The model under review builds one solid part; all positions refer to its coordinate system, in mm. Round coordinates to 2 decimals unless told otherwise and drop trailing zeros. Loops run counter-clockwise (first coordinate to the right, second up) from the corner with the lowest first, then second, coordinate; pieces in that order, holes last. Notation, with made-up numbers: M -13.5,-28.5 L 7.5,-28.5 A22 ccw 7.5,-14.5 Z; hole C -33,37.25 d5. An arc over 180 degrees is marked long. Return JSON: item names as keys, results as strings. Group by question number.
Q1. Consider section A-A (x = 0). State the section outline as (y, z) points (3 decimals).
Q2. Consider section B-B (z = 44.45). State the section outline as (x, y) points, and give its area (3 significant figures).
Q3. To check wall thickness, follow line 1 along Z through (x, y) = (0, 8); line 2 along X through (y, z) = (21.5, 44.45); line 3 along X through (y, z) = (16, 44). State the ranges of each line that lie inside material, in increasing order.
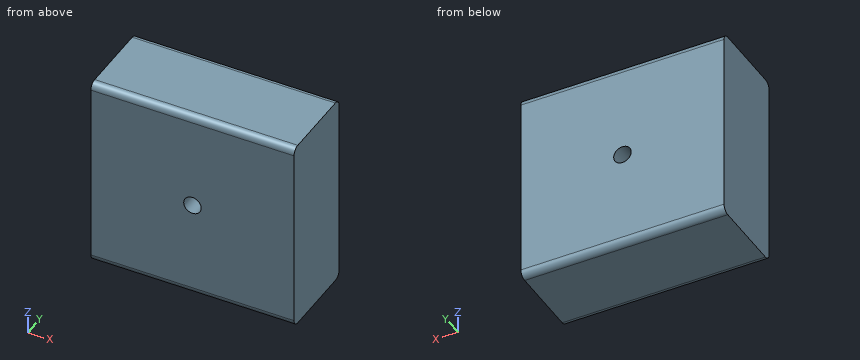
from build123d import *

# Parameters (mm, degrees)
SKETCH1_W                      = 92.075
SKETCH1_H                      = 38.1
BOSS_EXTRUDE1_DEPTH            = 88.9
FILLET1_R                      = 3.175
F_5_16_0_3125_DIAMETER_HOLE1_D = 7.9375


with BuildPart() as part:
    # Sketch1 → Boss-Extrude1 (new body)
    with BuildSketch(Plane.XY):
        with Locations((0, 19.05)):
            Rectangle(SKETCH1_W, SKETCH1_H)
    extrude(amount=BOSS_EXTRUDE1_DEPTH)

    # Fillet1
    fillet1_edges = [part.edges().sort_by_distance(p)[0] for p in [
        (0, 38.1, 88.9),
        (0, 38.1, 0),
        (0, 0, 0),
        (0, 0, 88.9),
    ]]
    fillet(fillet1_edges, radius=FILLET1_R)

    # 5/16 (0.3125) Diameter Hole1 (through all)
    with Locations(Plane(origin=(0, 38.1, 0), x_dir=(1, 0, 0), z_dir=(0, 1, 0))):
        with Locations((0, -44.45)):
            Hole(F_5_16_0_3125_DIAMETER_HOLE1_D / 2)


solid = part.part
Values:
{
 "1": {"outline": "M 0,3.175 A3.175 ccw 3.175,0 L 34.925,0 A3.175 ccw 38.1,3.175 L 38.1,40.481 L 0,40.481 Z; M 0,48.419 L 38.1,48.419 L 38.1,85.725 A3.175 ccw 34.925,88.9 L 3.175,88.9 A3.175 ccw 0,85.725 Z"},
 "2": {"outline": "M -46.04,0 L -3.97,0 L -3.97,38.1 L -46.04,38.1 Z; M 3.97,0 L 46.04,0 L 46.04,38.1 L 3.97,38.1 Z", "area": "3,210 mm2"},
 "3": {"line 1": "z = 0 to 40.48, 48.42 to 88.9", "line 2": "x = -46.04 to -3.97, 3.97 to 46.04", "line 3": "x = -46.04 to -3.94, 3.94 to 46.04"}
}
